For this review, take the finished solid that the model builds, in its own axes (mm). Face numbers are marked on the shaded views. A direction names the side the tool comes from. Give positions to 0.01 mm unless a question says otherwise; leave off trailing zeros. Loops run counter-clockwise (first coordinate to the right, second up) from the corner with the lowest first, then second, coordinate; pieces in that order, holes last. Notation, with made-up numbers: (6, 80) - (10, 80) arc R29 ccw to (10, 109) - close; hole circle Ø9 at (23, 76.5). An arc over 180 degrees is marked (long way). Put each result on its own line as item: value.
from build123d import *

# Parameters (mm, degrees)
F0_W      = 595.376
F0_H      = 335.788
F1_DEPTH  = 4.7625
F2_W      = 5.588
F2_H      = 324.612
F3_DEPTH  = 609.6
F4_W      = 595.376
F4_H      = 5.588
F6_DEPTH  = 600.075
F7_W      = 595.376
F7_H      = 5.588
F8_DEPTH  = 177.8
F10_DEPTH = 9.525
F11_R     = 3.175
F12_DEPTH = 9.525


with BuildPart() as f1:
    # F0 (on Front) → F1 (new body, symmetric)
    with BuildSketch(Plane.XZ):
        Rectangle(F0_W, F0_H)
    extrude(amount=F1_DEPTH, both=True)

    # F2 (on face) → F3 (join)
    with BuildSketch(Plane.XZ.offset(4.7625)):
        with Locations((-294.894, 0)):
            Rectangle(F2_W, F2_H)
        with Locations((294.894, 0)):
            Rectangle(F2_W, F2_H)
    extrude(amount=F3_DEPTH)

    # F4 (on face) → F6 (join, through all)
    with BuildSketch(Plane.XZ.offset(4.7625)):
        with Locations((0, 165.1)):
            Rectangle(F4_W, F4_H)
    extrude(amount=F6_DEPTH)

    # F7 (on face) → F8 (join)
    with BuildSketch(Plane(origin=(0, 4.7625, 0), x_dir=(-1, 0, 0), z_dir=(0, 1, 0))):
        with Locations((0, -165.1)):
            Rectangle(F7_W, F7_H)
    extrude(amount=-F8_DEPTH)

    # F9 (on face) → F10 (cut, through all)
    with BuildSketch(Plane(origin=(0, 4.7625, 0), x_dir=(-1, 0, 0), z_dir=(0, 1, 0))):
        with BuildLine():
            ThreePointArc((-246.888, 152.019), (-273.8287683632, 140.8597683632), (-284.988, 113.919))
            Line((-284.988, 113.919), (-284.988, -113.919))
            ThreePointArc((-284.988, -113.919), (-273.8287683632, -140.8597683632), (-246.888, -152.019))
            Line((-246.888, -152.019), (-246.888, 152.019))
        make_face()
        with BuildLine():
            Line((284.988, -113.919), (284.988, 113.919))
            ThreePointArc((284.988, 113.919), (273.8287683632, 140.8597683632), (246.888, 152.019))
            Line((246.888, 152.019), (246.888, -152.019))
            ThreePointArc((246.888, -152.019), (273.8287683632, -140.8597683632), (284.988, -113.919))
        make_face()
    extrude(amount=-F10_DEPTH, mode=Mode.SUBTRACT)

    # F11 (on face) → F12 (cut, through all)
    with BuildSketch(Plane(origin=(0, 4.7625, 0), x_dir=(-1, 0, 0), z_dir=(0, 1, 0))):
        with Locations((-216.2556, 144.7546)):
            Circle(F11_R)
        with Locations((-216.2556, -144.7546)):
            Circle(F11_R)
        with Locations((216.2556, 144.7546)):
            Circle(F11_R)
        with Locations((216.2556, -144.7546)):
            Circle(F11_R)
    extrude(amount=-F12_DEPTH, mode=Mode.SUBTRACT)


solid = f1.part
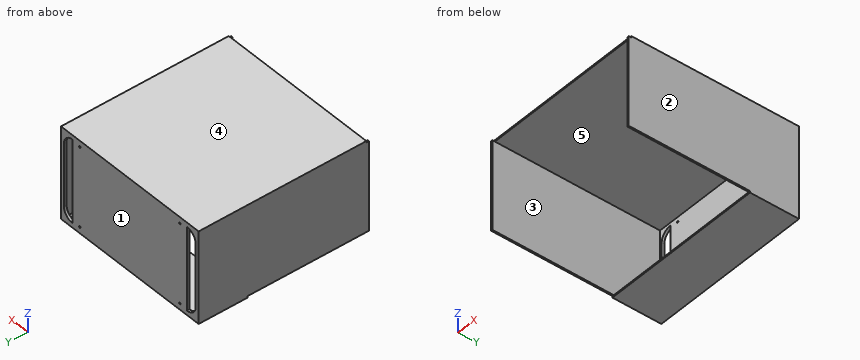
1) Take a section at A-A on z = 52.5. State the section outline as (x, y) points.
Geometry check:
outline: (-297.69, -614.36) - (-292.1, -614.36) - (-292.1, -4.76) - (-284.99, -4.76) - (-284.99, 4.76) - (-297.69, 4.76) - close; (-246.89, -4.76) - (246.89, -4.76) - (246.89, 4.76) - (-246.89, 4.76) - close; (284.99, -4.76) - (292.1, -4.76) - (292.1, -614.36) - (297.69, -614.36) - (297.69, 4.76) - (284.99, 4.76) - close
2) For the marked faces 4 and 5, list the 3-axis set-ups (+Z, -Z, +X, -X, +Y, -Y) from which the entire face can be reached by the end or side of a thin tool; tool diameter is ignored.
Geometry check:
face 4: +Z, +X, -X, +Y, -Y
face 5: -Y
3) Draft analysis for pull direction X (two halves, no side actions). For the marked faces 1, 2 and 3, state which applies: pulls with the +X half, pulls with the -X half, needs draft (parallel to the pull), parting line crosses it, or undercut.
Geometry check:
face 1: needs draft
face 2: pulls with the +X half
face 3: undercut
4) Insertion check: pin 1 Ø3 at (x, y) = (-295.5, -477.5) entering from -Z; pin 2 Ø12 at (x, z) = (207, 92) entering from -Y; pin 3 Ø1.7 at (x, y) = (-295.5, -611) entering from +Z. Each pin has a flat end and moves straight along its axis. Give the tip position at first contact, or say it passes through.
Geometry check:
pin 1: stops at z = -162.31
pin 2: stops at y = -4.76
pin 3: stops at z = 162.31
5) Take a section at B-B on y = -160. State the section outline as (x, z) points.
Geometry check:
outline: (-297.69, -167.89) - (297.69, -167.89) - (297.69, 167.89) - (-297.69, 167.89) - close; hole (-292.1, -162.31) - (292.1, -162.31) - (292.1, 162.31) - (-292.1, 162.31) - close
6) Wall thickness on line 1 (X direction, y = -369.5, z = -71); line 2 (Z direction, x = -52, y = -81.5); line 3 (Y direction, x = 26, z = 53): over which ranges is each line inside the solid? List them lowest first.
Geometry check:
line 1: x = -297.69 to -292.1, 292.1 to 297.69
line 2: z = -167.89 to -162.31, 162.31 to 167.89
line 3: y = -4.76 to 4.76
7) Take a section at C-C on x = -115. State the section outline as (y, z) points.
Geometry check:
outline: (-604.84, 162.31) - (-4.76, 162.31) - (-4.76, -162.31) - (-173.04, -162.31) - (-173.04, -167.89) - (4.76, -167.89) - (4.76, 167.89) - (-604.84, 167.89) - close
